Autodesk Inventor part; units mm, degrees
ref_plane "YZ Plane" through (0, 0, 0) normal (1, 0, 0) x (0, 1, 0)
ref_plane "XZ Plane" through (0, 0, 0) normal (0, 1, 0) x (-1, 0, 0)
ref_plane "XY Plane" through (0, 0, 0) normal (0, 0, 1) x (1, 0, 0)
sketch "Sketch1" plane through (0, 0, 0) normal (0, 0, 1) x (1, 0, 0)
  line L0 (-25.4072, 25.3665) -> (76.1928, 25.3665)
  line L1 (76.1928, 25.3665) -> (76.1928, -76.2335)
  line L2 (76.1928, -76.2335) -> (-25.4072, -76.2335)
  line L3 (-25.4072, -76.2335) -> (-25.4072, 25.3665)
  point P0 (0, 0)
  dimension "d0" = 101.6
  dimension "d1" = 101.6
extrude "Extrusion1" add sketch "Sketch1" along normal blind 0.7366
sketch "Sketch2" plane through (0, 0, 0.7366) normal (0, 0, 1) x (1, 0, 0)
  line L0 (-25.4072, 25.3665) -> (76.1928, -76.2335)
  line L1 (76.1928, 25.3665) -> (-25.4072, -76.2335)
  circle A0 centre (25.3928, -25.4335) radius 27.432
  point P0 (0, 0)
  dimension "d4" = 54.864
extrude "Extrusion2" cut sketch "Sketch2" against normal blind 0.7366
sketch "Sketch3" plane through (0, 0, 0.7366) normal (0, 0, 1) x (1, 0, 0)
  line L0 (-25.4072, -76.2335) -> (-25.4072, 25.3665)
  line L1 (-25.4072, 25.3665) -> (-25.4072, -25.4335)
  line L2 (-25.4072, -25.4335) -> (-25.4072, 19.4102)
  line L3 (-25.4072, 25.3665) -> (76.1928, -76.2335)
  line L4 (76.1928, 25.3665) -> (-25.4072, -76.2335)
  circle A0 centre (-19.4509, 19.4102) radius 1.9812
  point P0 (0, 0)
  dimension "d7" = 44.8437
  dimension "d8" = 3.9624
extrude "Extrusion3" cut sketch "Sketch3" against normal blind 0.7366 contours A0 L3 | L3 A0
sketch "Sketch4" plane through (0, 0, 0.7366) normal (0, 0, 1) x (1, 0, 0)
  line L0 (-25.4072, -76.2335) -> (76.1928, 25.3665)
  line L1 (-25.4072, 25.3665) -> (76.1928, -76.2335)
  circle A0 centre (70.2365, 19.4102) radius 1.9819
  circle A1 centre (70.2365, -70.2772) radius 1.983
  circle A2 centre (-19.4509, -70.2772) radius 1.9812
  point P0 (0, 0)
extrude "Extrusion4" cut sketch "Sketch4" against normal blind 0.7366
sketch "Sketch5" plane through (0, 0, 0.7366) normal (0, 0, 1) x (1, 0, 0)
  circle A0 centre (25.3928, -25.4335) radius 27.432
  circle A1 centre (25.3928, -25.4335) radius 29.972
  circle A2 centre (25.3928, -25.4335) radius 32.512
  point P0 (0, 0)
  dimension "d13" = 59.944
  dimension "d14" = 65.024
extrude "Extrusion5" add sketch "Sketch5" along normal blind 6.6548 contours A2
fillet "Fillet1" radius 3.175 4 edges at (-25.4072, 25.3665, 0.3683) (76.1928, 25.3665, 0.3683) (76.1928, -76.2335, 0.3683) (-25.4072, -76.2335, 0.3683)
sketch "Sketch6" plane through (25.3928, -25.4335, 7.3914) normal (0, 0, 1) x (1, 0, 0)
  circle A0 centre (0, 0) radius 29.972
  circle A1 centre (0, 0) radius 32.512
  point P0 (-25.3928, 25.4335)
extrude "Extrusion6" cut sketch "Sketch6" against normal blind 3.3274
sketch "Sketch7" plane through (25.3928, -25.4335, 0.7366) normal (0, 0, 1) x (1, 0, 0)
  circle A0 centre (0, 0) radius 29.972
  circle A1 centre (0, 0) radius 27.432
  point P0 (-25.3928, 25.4335)
extrude "Extrusion7" add sketch "Sketch7" along normal blind 3.3274
sketch "Sketch8" plane through (0, 0, 0.7366) normal (0, 0, 1) x (1, 0, 0)
  circle A0 centre (-19.4509, 19.4102) radius 1.9812
  circle A1 centre (70.2365, -70.2772) radius 1.983
  circle A2 centre (-19.4509, -70.2772) radius 1.9812
  circle A3 centre (70.2365, 19.4102) radius 1.9819
  line L0 (-19.4509, 19.4102) -> (70.2365, -70.2772)
  line L1 (-19.4509, -70.2772) -> (70.2365, 19.4102)
  line L2 (-25.4072, 25.3665) -> (76.1928, 25.3665)
  line L3 (76.1928, 25.3665) -> (76.1928, -76.2335)
  line L4 (76.1928, -76.2335) -> (-25.4072, -76.2335)
  line L5 (-25.4072, -76.2335) -> (-25.4072, 25.3665)
  line L6 (-25.4072, 25.3665) -> (-25.4072, -25.4335)
  line L7 (-25.4072, -25.4335) -> (-25.4072, 15.0541)
  circle A4 centre (-15.0948, 15.0541) radius 1.9812
  circle A5 centre (65.8804, 15.0541) radius 1.9816
  circle A6 centre (65.8804, -65.9211) radius 1.9817
  circle A7 centre (-15.0948, -65.9211) radius 1.9817
  point P0 (0, 0)
  dimension "d22" = 40.4876
  dimension "d23" = 3.9624
extrude "Extrusion8" cut sketch "Sketch8" against normal blind 3.3274 contours A5 L1 | L1 A5 | A6 L0 | L0 A6 | A7 L1 | L1 A7 | A4 L0 | L0 A4
properties part number "3"
Design review of the part built by this model. Coordinates are the model's own, in mm. A direction names the side the tool comes from. Round coordinates to 2 decimals unless told otherwise and drop trailing zeros. Loops run counter-clockwise (first coordinate to the right, second up) from the corner with the lowest first, then second, coordinate; pieces in that order, holes last. Notation, with made-up numbers: (5.25, 61) -> (47.25, 61) arc R10 ccw to (47.25, 71) -> close; hole circle Ø8 at (10.25, 45.5). An arc over 180 degrees is marked (long way). Use one line per item in the form item = value. Start each with the question number.
Q1. We need section C-C on z = 2.4. Give the boundary of the cut face in (x, y).
Q2. Wall thickness on line 1 along X through (y, z) = (14, 0.2); line 2 along Y through (x, z) = (68.5, 0.6); line 3 along X through (y, z) = (-38, 2.85): over which ranges is each line inside the solid? List them lowest first. Write a range as [from, to].
Q3. Machinability: for faces 1 (the face through (2, -2, 0)), 2 (the face through (2, -2, 0.737)), which of the approach directions +Z, -Z, +X, -X, +Y, -Y give a long, thin tool a straight path to every point of the face, cutting with its end or side? Answer none if there is none.
Q4. For pin 1 Ø1 at (x, z) = (21.5, 3.5) entering from +Y; pin 2 Ø5 at (x, y) = (-19.45, 19.41) entering from +Z; pin 3 Ø1 at (x, z) = (56, 2) entering from -Y, all flat-tipped, find the tip position at first contact; note any pin that passes through.
Q5. Draft analysis for pull direction Y (two halves, no side actions). For faces 3 (the face through (8, -47, 4.064)), 4 (the face through (56.403, -35.199, 2.377)), 5 (the face through (68.664, 18.204, 0.373)), state which applies: +Y half, -Y half, draft (parallel to the pull), parting line (faces both ways), or undercut.
Q6. We need section B-B on x = 17.5. Give the boundary of the cut face in (y, z).
Q7. We need section A-A on y = -34. Give the boundary of the cut face in (x, z), then the cut area to 3 significant figures.
Calculated:
q1.outline = circle Ø65.02 at (25.39, -25.43); hole circle Ø54.86 at (25.39, -25.43)
q2.line_1 = [-25.41, -16.77], [-13.42, 64.2], [67.56, 76.19]
q2.line_2 = [-76.23, -71.23], [-69.32, 18.45], [20.37, 25.37]
q2.line_3 = [-4.59, 1.01], [49.78, 55.38]
q3.face_1 = -Z, +X, -X, +Y, -Y
q3.face_2 = +Z
q4.pin_1 = 6.9
q4.pin_2 = 0.74
q4.pin_3 = -37.7
q5.face_3 = draft
q5.face_4 = parting line
q5.face_5 = undercut
q6.outline = (-76.23, 0) -> (-51.71, 0) -> (-51.71, 4.06) -> (-56.97, 4.06) -> (-56.97, 0.74) -> (-76.23, 0.74) -> close; (0.84, 0) -> (25.37, 0) -> (25.37, 0.74) -> (6.11, 0.74) -> (6.11, 4.06) -> (0.84, 4.06) -> close
q7.outline = (-25.41, 0) -> (-0.67, 0) -> (-0.67, 4.06) -> (-5.97, 4.06) -> (-5.97, 0.74) -> (-25.41, 0.74) -> close; (51.45, 0) -> (76.19, 0) -> (76.19, 0.74) -> (56.76, 0.74) -> (56.76, 4.06) -> (51.45, 4.06) -> close
q7.area = 71.7 mm²
